from build123d import *

# Parameters (mm, degrees)
SKETCH_1_W                   = 18.65
SKETCH_1_H                   = 32
EXTRUDE_1_DEPTH              = 20
SKETCH_2_W                   = 10.75
SKETCH_2_H                   = 32
CUT_EXTRUDE_2_DEPTH          = 17
CUT_EXTRUDE_3_REACH          = 22
SKETCH_4_W                   = 10.65
SKETCH_4_H                   = 8
FILLET_1_R                   = 2
HOLE_WIZARD_M3_4_D           = 3.4
HOLE_WIZARD_M3_4_DEPTH       = 3.95
HOLE_WIZARD_M3_4_CSINK_D     = 3.45
HOLE_WIZARD_M3_4_CSINK_ANGLE = 92
SKETCH_18_W                  = 13.75
SKETCH_18_H                  = 5
EXTRUDE_2_DEPTH              = 16
SKETCH_19_W                  = 13.75
SKETCH_19_H                  = 3
EXTRUDE_3_DEPTH              = 18
CUT_EXTRUDE_4_REACH          = 38
SKETCH_20_R                  = 2.35


with BuildPart() as part:
    # 스케치1 → 보스-돌출1 (new body)
    with BuildSketch(Plane.XY):
        Rectangle(SKETCH_1_W, SKETCH_1_H)
    extrude(amount=-EXTRUDE_1_DEPTH)

    # 스케치2 → 컷-돌출2 (cut)
    with BuildSketch(Plane(origin=(0, 0, -20), x_dir=(-1, 0, 0), z_dir=(0, 0, -1))):
        Rectangle(SKETCH_2_W, SKETCH_2_H)
    extrude(amount=-CUT_EXTRUDE_2_DEPTH, mode=Mode.SUBTRACT)

    # 스케치4 → 컷-돌출3 (cut, up to next)
    with BuildSketch(Plane.XY, mode=Mode.PRIVATE) as cut_extrude_3_sk1:
        with Locations((0, 12)):
            Rectangle(SKETCH_4_W, SKETCH_4_H)
    cut_extrude_3_tool1 = extrude(cut_extrude_3_sk1.sketch, amount=-CUT_EXTRUDE_3_REACH, mode=Mode.PRIVATE) & part.part
    add(cut_extrude_3_tool1.solids().sort_by_distance((0, 12, 0))[0], mode=Mode.SUBTRACT)

    # 필렛1
    fillet_1_edges = [part.edges().sort_by_distance(p)[0] for p in [
        (-7.35, 16, -20),
        (7.35, 16, -20),
    ]]
    fillet(fillet_1_edges, radius=FILLET_1_R)

    # M3 여유 구멍4
    with Locations(Plane(origin=(9.325, 0, 0), x_dir=(0, 0, -1), z_dir=(1, 0, 0))):
        with Locations((17, 13), (17, -12.4), (38.233038072, 15.712174446)):
            CounterSinkHole(HOLE_WIZARD_M3_4_D / 2, HOLE_WIZARD_M3_4_CSINK_D / 2, depth=HOLE_WIZARD_M3_4_DEPTH, counter_sink_angle=HOLE_WIZARD_M3_4_CSINK_ANGLE)

    # 스케치18 → 보스-돌출2 (add)
    with BuildSketch(Plane.XY):
        with Locations((0, 3.5)):
            Rectangle(SKETCH_18_W, SKETCH_18_H)
    extrude(amount=EXTRUDE_2_DEPTH)

    # 스케치19 → 보스-돌출3 (add)
    with BuildSketch(Plane.XZ.offset(-1)):
        with Locations((0, 14.5)):
            Rectangle(SKETCH_19_W, SKETCH_19_H)
    extrude(amount=EXTRUDE_3_DEPTH)

    # 스케치20 → 컷-돌출4 (cut, up to next)
    with BuildSketch(Plane.XY.offset(16), mode=Mode.PRIVATE) as cut_extrude_4_sk1:
        with Locations((0, -9.320578261)):
            Circle(SKETCH_20_R)
    cut_extrude_4_tool1 = extrude(cut_extrude_4_sk1.sketch, amount=-CUT_EXTRUDE_4_REACH, mode=Mode.PRIVATE) & part.part
    add(cut_extrude_4_tool1.solids().sort_by_distance((0, -9.320578, 16))[0], mode=Mode.SUBTRACT)


solid = part.part
Read the model definition and answer for the solid it produces. Units are mm, in the model's axes. A direction names the side the tool comes from. Round coordinates to 2 decimals unless told otherwise and drop trailing zeros. Loops run counter-clockwise (first coordinate to the right, second up) from the corner with the lowest first, then second, coordinate; pieces in that order, holes last.
Q1. Each of these flat-tipped pins is pushed along its axis until it touches: pin 1 (3 mm diameter, centred on x = 3, z = -4, fed in from -Y); pin 2 (5.5 mm diameter, centred on x = 1.5, y = 6, fed in from -Z); pin 3 (6.5 mm diameter, centred on x = -1.5, z = 4.5, fed in from -Y). Where does it stop, or does it pass through?
Q2. Section C-C on x = 0 is taken. Write down the section's boundary in (y, z), and give its area (3 significant figures).
Q3. Determine the mould class of faces 4 (the face through (-0.31, -6.99, 14.52)), 5 (the face through (7, 16, -9)), 6 (the face through (-9.325, 0, -10)) for opening direction X: released by +X, released by -X, zero draft, split by the parting line, or undercut.
Q4. Which of the six approach directions +Z, -Z, +X, -X, +Y, -Y give full straight-line access (tool end or side, diameter ignored) to faces 1 (the face through (5.325, 12, -1)), 2 (the face through (7.31, 13.51, -15.38)), 3 (the face through (0, -6, 13))?
Q5. Section A-A on z = -17 is taken. Write down the section's boundary in (x, y) (3 decimals), and give its area (3 significant figures).
Q6. Section B-B on y = 13 is taken. Write down the section's boundary in (x, z) (3 decimals), and give its area (3 significant figures).
Q7. Section D-D on y = 9 is taken. Write down the section's boundary in (x, z) (3 decimals).
Q8. Consider probe 1 along Y at (x, z) = (8.45, -17); probe 2 along Z at (x, y) = (6.35, -12.4); probe 3 along Z at (x, y) = (0.25, -0.5). Determine where each line is inside the solid, lowest interval first.
Output:
1. pin 1: stops at y = -16
1. pin 2: stops at z = -3
1. pin 3: stops at y = 1
2. outline: (-17, 13) - (-11.67, 13) - (-11.67, 16) - (-17, 16) - close; (-16, -3) - (8, -3) - (8, 0) - (6, 0) - (6, 16) - (-6.97, 16) - (-6.97, 13) - (1, 13) - (1, 0) - (-16, 0) - close
2. area: 192 mm2
3. face 4: undercut
3. face 5: zero draft
3. face 6: released by -X
4. face 1: +Z, -Z, +Y
4. face 2: +X
4. face 3: +X, -X, -Y
5. outline: (-9.325, -16) - (-5.375, -16) - (-5.375, 16) - (-9.325, 16) - close; (5.375, -16) - (9.325, -16) - (9.325, -14.125) - (9.301, -14.1) - (5.375, -14.1) - close; (5.375, -10.7) - (9.301, -10.7) - (9.325, -10.675) - (9.325, 11.275) - (9.301, 11.3) - (5.375, 11.3) - close; (5.375, 14.7) - (9.301, 14.7) - (9.325, 14.725) - (9.325, 16) - (5.375, 16) - close
5. area: 226 mm2
6. outline: (-9.325, -20) - (-5.375, -20) - (-5.375, -3) - (-5.325, -3) - (-5.325, 0) - (-9.325, 0) - close; (5.325, -3) - (5.375, -3) - (5.375, -15.3) - (9.301, -15.3) - (9.325, -15.275) - (9.325, 0) - (5.325, 0) - close; (5.375, -20) - (9.325, -20) - (9.325, -18.725) - (9.301, -18.7) - (5.375, -18.7) - close
6. area: 145 mm2
7. outline: (-9.325, -20) - (-5.375, -20) - (-5.375, -3) - (-5.325, -3) - (-5.325, 0) - (-9.325, 0) - close; (5.325, -3) - (5.375, -3) - (5.375, -20) - (9.325, -20) - (9.325, 0) - (5.325, 0) - close
8. probe 1: y = -16 to -14.1, -10.7 to 11.3, 14.7 to 16
8. probe 2: z = -20 to -18.7, -15.3 to 0, 13 to 16
8. probe 3: z = -3 to 0, 13 to 16
